Check sheet for the modelled part. Datum: model origin and axes. Units: mm. A direction names the side the tool comes from. Give positions to 0.01 mm unless a question says otherwise; leave off trailing zeros. Loops run counter-clockwise (first coordinate to the right, second up) from the corner with the lowest first, then second, coordinate; pieces in that order, holes last. Notation, with made-up numbers: (-16, 20) - (43, 20) arc R10 cw to (43, 38) - close; hole circle Ø2 at (-27, 8.25). An arc over 180 degrees is marked (long way). Use one line per item in the form item = value.
from build123d import *

# Parameters (mm, degrees)
BOSS_EXTRUDE1_DEPTH                              = 200
CUT_EXTRUDE1_DEPTH                               = 201
F_0_4_0_4_DIAMETER_HOLE1_D                       = 0.4
F_0_4_0_4_DIAMETER_HOLE1_DEPTH                   = 200
CBORE_FOR_M4_HEX_HEAD_MACHINE_SCREW1_D           = 4.5
CBORE_FOR_M4_HEX_HEAD_MACHINE_SCREW1_DEPTH       = 4.1
CBORE_FOR_M4_HEX_HEAD_MACHINE_SCREW1_CBORE_D     = 8.5
CBORE_FOR_M4_HEX_HEAD_MACHINE_SCREW1_CBORE_DEPTH = 3.1
FILLET1_R                                        = 0.2
FILLET2_R                                        = 0.5
FILLET3_R                                        = 1


with BuildPart() as part:
    # Sketch1 → Boss-Extrude1 (new body)
    with BuildSketch(Plane(origin=(0, 300, 0), x_dir=(1, 0, 0), z_dir=(0, 1, 0))):
        with BuildLine():
            Line((-13.5, -3), (-13.5, -8.7))
            Line((-13.5, -8.7), (13.5, -8.7))
            Line((13.5, -8.7), (13.5, -3))
            Line((13.5, -3), (7.8, -3))
            ThreePointArc((7.8, -3), (7.05, -2.25), (7.8, -1.5))
            Line((7.8, -1.5), (11, -1.5))
            Line((11, -1.5), (11, 0))
            Line((11, 0), (-11, 0))
            Line((-11, 0), (-11, -1.5))
            Line((-11, -1.5), (-7.8, -1.5))
            ThreePointArc((-7.8, -1.5), (-7.05, -2.25), (-7.8, -3))
            Line((-7.8, -3), (-13.5, -3))
        make_face()
    extrude(amount=-BOSS_EXTRUDE1_DEPTH)

    # Sketch2 → Cut-Extrude1 (cut, through all)
    with BuildSketch(Plane.XZ.offset(-100)):
        Polygon((8.75, 8.7), (-8.75, 8.7), (-8.75, 7.6), (-12, 7.6), (-12, 4.1), (12, 4.1), (12, 7.6), (8.75, 7.6), align=None)
    extrude(amount=-CUT_EXTRUDE1_DEPTH, mode=Mode.SUBTRACT)

    # Ø0.4 (0.4) Diameter Hole1
    with Locations(Plane(origin=(0, 300, 0), x_dir=(1, 0, 0), z_dir=(0, 1, 0))):
        with Locations((-7.75, -4.1), (7.75, -4.1)):
            Hole(F_0_4_0_4_DIAMETER_HOLE1_D / 2, depth=F_0_4_0_4_DIAMETER_HOLE1_DEPTH)

    # CBORE for M4 Hex Head Machine Screw1
    with Locations(Plane.XY.offset(4.1)):
        with Locations((0, 260), (0, 200), (0, 140), (0, 80), (0, 20)):
            CounterBoreHole(CBORE_FOR_M4_HEX_HEAD_MACHINE_SCREW1_D / 2, CBORE_FOR_M4_HEX_HEAD_MACHINE_SCREW1_CBORE_D / 2, CBORE_FOR_M4_HEX_HEAD_MACHINE_SCREW1_CBORE_DEPTH, depth=CBORE_FOR_M4_HEX_HEAD_MACHINE_SCREW1_DEPTH)

    # Fillet1
    fillet1_edges = [part.edges().sort_by_distance(p)[0] for p in [
        (-11, 200, 1.5),
        (11, 200, 1.5),
    ]]
    fillet(fillet1_edges, radius=FILLET1_R)

    # Fillet2
    fillet2_edges = [part.edges().sort_by_distance(p)[0] for p in [
        (12, 200, 7.6),
        (12, 200, 4.1),
        (-12, 200, 4.1),
        (-12, 200, 7.6),
    ]]
    fillet(fillet2_edges, radius=FILLET2_R)

    # Fillet3
    fillet3_edges = [part.edges().sort_by_distance(p)[0] for p in [
        (13.5, 200, 3),
        (13.5, 200, 8.7),
        (-13.5, 200, 8.7),
        (-13.5, 200, 3),
    ]]
    fillet(fillet3_edges, radius=FILLET3_R)


solid = part.part
Item 1: Thickness scan on L1, parallel to Y at x = -0.5, z = 1.5; L2, parallel to X at y = 153.5, z = 4; L3, parallel to Z at x = 11.25, y = 171.5. Record the ranges inside material, lowest first.
Answer block:
L1 = 100 to 135.78, 144.22 to 195.78, 204.22 to 255.78, 264.22 to 300
L2 = -13.5 to -7.92, -7.58 to 7.58, 7.92 to 13.5
L3 = 3 to 4.1, 7.6 to 8.7
Item 2: Access from +Z, -Z, +X, -X, +Y, -Y to the whole of each face (thin tool, end or side, straight path). Record for faces 1 (the face through (10, 199, 4.1)), 2 (the face through (2, 138, 1)), 3 (the face through (-5, 199, 4.1)), 4 (the face through (0.488, 137.804, 0.493)).
Answer block:
face_1 = +Y, -Y
face_2 = +Z
face_3 = +Z, +Y, -Y
face_4 = +Z, -Z
Item 3: Mould release check, pull along Z, two halves, no side actions. Record for faces 5 (the face through (13.5, 201, 6)), 6 (the face through (2, 258, 1)), 7 (the face through (10, 201, 3)): released by +Z, released by -Z, zero draft, split by the parting line, or undercut.
Answer block:
face_5 = zero draft
face_6 = released by +Z
face_7 = undercut
Item 4: Gauge pin test, flat ends, axial feed: P1, Ø9.5, axis at x = 1, y = 259, coming from the +Z side; P2, Ø6, axis at x = 0, y = 260, coming from the +Z side. Record the tip position at first contact, or that the pin passes through.
Answer block:
P1 = 4.1
P2 = 1
Item 5: Section check A-A on x = 0. Record the boundary of the cut face in (y, z).
Answer block:
outline = (100, 0) - (137.75, 0) - (137.75, 1) - (135.75, 1) - (135.75, 4.1) - (100, 4.1) - close; (142.25, 0) - (197.75, 0) - (197.75, 1) - (195.75, 1) - (195.75, 4.1) - (144.25, 4.1) - (144.25, 1) - (142.25, 1) - close; (202.25, 0) - (257.75, 0) - (257.75, 1) - (255.75, 1) - (255.75, 4.1) - (204.25, 4.1) - (204.25, 1) - (202.25, 1) - close; (262.25, 0) - (300, 0) - (300, 4.1) - (264.25, 4.1) - (264.25, 1) - (262.25, 1) - close
